from build123d import *

# Parameters (mm, degrees)
SKETCH_R        = 4
SKETCH_R_2      = 2.5
SKETCH_R_3      = 1.5
SKETCH_R_4      = 2.6
PAD_DEPTH       = 4
SKETCH006_W     = 88
SKETCH006_H     = 10
PAD001_DEPTH    = 4
SKETCH007_R     = 2.5
SKETCH007_R_2   = 1.5
POCKET_DEPTH    = 8.001
FILLET_R        = 10
FILLET001_R     = 10
FILLET002_R     = 4
FILLET003_R     = 4
CHAMFER_SIZE    = 2
CHAMFER001_SIZE = 2
CHAMFER002_SIZE = 2


with BuildPart() as part:
    # Sketch → Pad (new body)
    with BuildSketch(Plane.XY):
        Polygon((80, 5), (98, 17.603736), (98, 22), (118, 22), (118, -22), (98, -22), (98, -17.603736), (80, -5), (28, -5), (10, -17.603736), (10, -22), (-10, -22), (-10, 22), (10, 22), (10, 17.603736), (28, 5), align=None)
        with Locations((108, 0)):
            Circle(SKETCH_R, mode=Mode.SUBTRACT)
        with Locations((39, 0)):
            Circle(SKETCH_R_2, mode=Mode.SUBTRACT)
        with Locations((79, 0)):
            Circle(SKETCH_R_2, mode=Mode.SUBTRACT)
        with Locations((72.5, 0)):
            Circle(SKETCH_R_3, mode=Mode.SUBTRACT)
        with Locations((68.5, 0)):
            Circle(SKETCH_R_3, mode=Mode.SUBTRACT)
        with Locations((108, 16)):
            Circle(SKETCH_R_4, mode=Mode.SUBTRACT)
        with Locations((108, -16)):
            Circle(SKETCH_R_4, mode=Mode.SUBTRACT)
        with Locations((0, 16)):
            Circle(SKETCH_R_4, mode=Mode.SUBTRACT)
        Circle(SKETCH_R, mode=Mode.SUBTRACT)
        with Locations((0, -16)):
            Circle(SKETCH_R_4, mode=Mode.SUBTRACT)
    extrude(amount=PAD_DEPTH)

    # Sketch006 (on Face28 of Pad) → Pad001 (join)
    with BuildSketch(Plane.XY.offset(4)):
        with Locations((54, 0)):
            Rectangle(SKETCH006_W, SKETCH006_H)
    extrude(amount=PAD001_DEPTH)

    # Sketch007 → Pocket (cut, through all)
    with BuildSketch(Plane.XY):
        with Locations((39, 0)):
            Circle(SKETCH007_R)
        with Locations((79, 0)):
            Circle(SKETCH007_R)
        with Locations((72.5, 0)):
            Circle(SKETCH007_R_2)
        with Locations((68.5, 0)):
            Circle(SKETCH007_R_2)
    extrude(amount=POCKET_DEPTH, mode=Mode.SUBTRACT)

    # Fillet
    fillet_edges = [part.edges().sort_by_distance(p)[0] for p in [
        (-10, -22, 2),
        (-10, 22, 2),
    ]]
    fillet(fillet_edges, radius=FILLET_R)

    # Fillet001
    fillet001_edges = [part.edges().sort_by_distance(p)[0] for p in [
        (118, 22, 2),
        (118, -22, 2),
    ]]
    fillet(fillet001_edges, radius=FILLET001_R)

    # Fillet002
    fillet002_edges = [part.edges().sort_by_distance(p)[0] for p in [
        (10, 22, 2),
        (98, 22, 2),
    ]]
    fillet(fillet002_edges, radius=FILLET002_R)

    # Fillet003
    fillet003_edges = [part.edges().sort_by_distance(p)[0] for p in [
        (10, -22, 2),
        (98, -22, 2),
    ]]
    fillet(fillet003_edges, radius=FILLET003_R)

    # Chamfer
    chamfer_edges = [part.edges().sort_by_distance(p)[0] for p in [
        (89, -5, 4),
    ]]
    chamfer(chamfer_edges, length=CHAMFER_SIZE)

    # Chamfer001
    chamfer001_edges = [part.edges().sort_by_distance(p)[0] for p in [
        (19, -5, 4),
    ]]
    chamfer(chamfer001_edges, length=CHAMFER001_SIZE)

    # Chamfer002
    chamfer002_edges = [part.edges().sort_by_distance(p)[0] for p in [
        (19, 5, 4),
        (89, 5, 4),
    ]]
    chamfer(chamfer002_edges, length=CHAMFER002_SIZE)


solid = part.part
Verification items for the finished model (mm, model axes). A direction names the side the tool comes from. Coordinates: 2 decimals unless noted, no trailing zeros. Loops run counter-clockwise (first coordinate to the right, second up) from the corner with the lowest first, then second, coordinate; pieces in that order, holes last. Notation, with made-up numbers: (84.5, 61) -> (93.5, 61) arc R27 cw to (93.5, 84) -> close; hole circle Ø2 at (37, 55.25). An arc over 180 degrees is marked (long way). Answer as CSV lines item,"result".
1) Tool access check on faces 4 (the flat face through (53, 5, 5)), 5 (the flat face through (98, 0, 6)), 6 (the flat face through (18.874, 11.39, 2.291)), 7 (the flat face through (89.126, -11.39, 2.291)), 8 (the flat face through (55, 0, 0)). Record the directions out of +Z, -Z, +X, -X, +Y, -Y that give a thin tool (end or side, any length) a straight path to the whole face; none if there is none.
Found:
face 4,"+Z, +Y"
face 5,"+Z, +X, +Y, -Y"
face 6,"+Z, -Z, +Y"
face 7,"+Z, -Z, -Y"
face 8,"-Z, +X, -X, +Y, -Y"
2) Cross-section at D-D, the plane x = 89.5. Record the cut outline in (y, z).
Found:
outline,"(-11.65, 0) -> (11.65, 0) -> (11.65, 4) -> (7, 4) -> (5, 6) -> (5, 8) -> (-5, 8) -> (-5, 6) -> (-7, 4) -> (-11.65, 4) -> close"
3) Cross-section at C-C, the plane y = 10.5. Record the cut outline in (x, z).
Found:
outline,"(-10, 0) -> (20.15, 0) -> (20.15, 4) -> (-10, 4) -> close; (87.85, 0) -> (118, 0) -> (118, 4) -> (87.85, 4) -> close"
4) Thickness scan on L1, parallel to Y at x = 108, z = 2; L2, parallel to X at y = 17.5, z = 0.5; L3, parallel to Y at x = 59.5, z = 7.5. Record the ranges inside material, lowest first. Write a range as from..to.
Found:
L1,"y = -22..-18.6, -13.4..-4, 4..13.4, 18.6..22"
L2,"x = -8.35..-2.12, 2.12..10.15, 97.85..105.88, 110.12..116.35"
L3,"y = -5..5"
5) Depth check by flat-ended pin: pin 1 (1.5 mm diameter, centred on x = 14.5, y = -10, fed in from +Z); pin 2 (3 mm diameter, centred on y = -2, z = 6, fed in from +X); pin 3 (1.5 mm diameter, centred on x = 26.5, z = 4.5, fed in from -Y). Enter the tip coordinate at first touch or a pass-through.
Found:
pin 1,"stops at z = 4"
pin 2,"stops at x = 98"
pin 3,"stops at y = -6.57"
6) Cross-section at A-A, the plane y = 0. Count the separate pieces of the cut face and the enclosed holes in it, then the cut area to 3 significant figures.
Found:
separate pieces,"7"
enclosed holes,"0"
area,"672 mm2"
7) Release check for a two-part mould opening along Y. For faces 1 (the cylindrical face through (110.48, -15.22, 1.97)), 2 (the flat face through (105, 22, 2)), 3 (the cylindrical face through (115.15, -18.99, 2.03)) record: +Y half, -Y half, draft (parallel to the pull), parting line (faces both ways), or undercut.
Found:
face 1,"undercut"
face 2,"+Y half"
face 3,"-Y half"
8) Cross-section at B-B, the plane x = 39. Record the cut outline in (y, z), then the cut area to 3 significant figures.
Found:
outline,"(-5, 0) -> (-2.5, 0) -> (-2.5, 8) -> (-5, 8) -> close; (2.5, 0) -> (5, 0) -> (5, 8) -> (2.5, 8) -> close"
area,"40.0 mm2"
